```python
from build123d import *

# Parameters (mm, degrees)
F1_DEPTH = 26.9748
F2_W     = 38.1
F2_H     = 9.779
F3_DEPTH = 9.525
F4_W     = 18.923
F4_H     = 19.05
F5_DEPTH = 63.5
F6_R     = 2.794
F7_DEPTH = 2.54


with BuildPart() as f1:
    # F0 (on Top) → F1 (new body)
    with BuildSketch(Plane.XY):
        Polygon((0, 38.1), (0, 0), (9.525, 0), (13.945783, 3.417956), (28.448, 38.1), align=None)
    extrude(amount=F1_DEPTH)

    # F2 (on face) → F3 (cut)
    with BuildSketch(Plane(origin=(0, 0, 0), x_dir=(0, -1, 0), z_dir=(-1, 0, 0))):
        with Locations((-19.05, 14.1605)):
            Rectangle(F2_W, F2_H)
    extrude(amount=-F3_DEPTH, mode=Mode.SUBTRACT)

    # F4 (on face) → F5 (join)
    with BuildSketch(Plane(origin=(0, 38.1, 0), x_dir=(-1, 0, 0), z_dir=(0, 1, 0))):
        with Locations((-18.9865, 9.525)):
            Rectangle(F4_W, F4_H)
    extrude(amount=F5_DEPTH)

    # F6 (on face) → F7 (cut)
    with BuildSketch(Plane.XY.offset(26.9748)):
        with Locations((4.7498, 31.75)):
            Circle(F6_R)
        with Locations((4.7498, 19.05)):
            Circle(F6_R)
        with Locations((4.7498, 6.35)):
            Circle(F6_R)
    extrude(amount=-F7_DEPTH, mode=Mode.SUBTRACT)


solid = f1.part
```
Read the model definition and answer for the solid it produces. Units are mm, in the model's axes. A direction names the side the tool comes from. Give positions to 0.01 mm unless a question says otherwise; leave off trailing zeros. Loops run counter-clockwise (first coordinate to the right, second up) from the corner with the lowest first, then second, coordinate; pieces in that order, holes last.
Item 1: The part is cut by section A-A (x = 8.5). Write down the section's boundary in (y, z).
Item 2: Each of these flat-tipped pins is pushed along its axis until it touches: pin 1 Ø1 at (x, y) = (20, 81.5) entering from +Z; pin 2 Ø1.5 at (y, z) = (63, 6.5) entering from -X (3 decimals); pin 3 Ø2 at (x, z) = (12.5, 21) entering from +Y. Where does it stop, or does it pass through?
Item 3: The part is cut by section B-B (z = 11.25). Write down the section's boundary in (x, y) (3 decimals).
Item 4: For faces 1 (the flat face through (21.095, 20.516, 13.299)), 2 (the cylindrical face through (2.69, 8.24, 25.72)), 3 (the flat face through (5, 19, 9.271)), determine the directions among +Z, -Z, +X, -X, +Y, -Y from which every point of the face is accessible in a straight line to the end or side of a thin tool.
Item 5: Find the intervals of material crossed by line 1 along X through (y, z) = (90.5, 13.25) (3 decimals); line 2 along Z through (x, y) = (8.5, 26); line 3 along Z through (x, y) = (14.25, 78), in increasing order.
Item 6: The part is cut by section C-C (y = 31.75). Write down the section's boundary in (x, z) (3 decimals).
Item 7: The mould has two halves that part along Y. Classify faces 4 (the flat face through (14, 38.1, 23)), 5 (the flat face through (5, 32, 24.435)), 6 (the flat face through (19, 69, 19.05)): released by +Y, released by -Y, zero draft, split by the parting line, or undercut.
Item 8: The part is cut by section D-D (x = 3). Write down the section's boundary in (y, z).
Taken from the geometry:
1. outline: (0, 0) - (38.1, 0) - (38.1, 9.27) - (0, 9.27) - close; (0, 19.05) - (38.1, 19.05) - (38.1, 26.97) - (0, 26.97) - close
2. pin 1: stops at z = 19.05
2. pin 2: stops at x = 9.525
2. pin 3: stops at y = 38.1
3. outline: (9.525, 0) - (13.946, 3.418) - (28.448, 38.1) - (28.448, 101.6) - (9.525, 101.6) - close
4. face 1: +Z, -Z, +X, -Y
4. face 2: +Z
4. face 3: -X, +Y, -Y
5. line 1: x = 9.525 to 28.448
5. line 2: z = 0 to 9.27, 19.05 to 26.97
5. line 3: z = 0 to 19.05
6. outline: (0, 0) - (25.793, 0) - (25.793, 26.975) - (7.544, 26.975) - (7.544, 24.435) - (1.956, 24.435) - (1.956, 26.975) - (0, 26.975) - (0, 19.05) - (9.525, 19.05) - (9.525, 9.271) - (0, 9.271) - close
7. face 4: released by +Y
7. face 5: undercut
7. face 6: zero draft
8. outline: (0, 0) - (38.1, 0) - (38.1, 9.27) - (0, 9.27) - close; (0, 19.05) - (38.1, 19.05) - (38.1, 26.97) - (33.93, 26.97) - (33.93, 24.43) - (29.57, 24.43) - (29.57, 26.97) - (21.23, 26.97) - (21.23, 24.43) - (16.87, 24.43) - (16.87, 26.97) - (8.53, 26.97) - (8.53, 24.43) - (4.17, 24.43) - (4.17, 26.97) - (0, 26.97) - close
